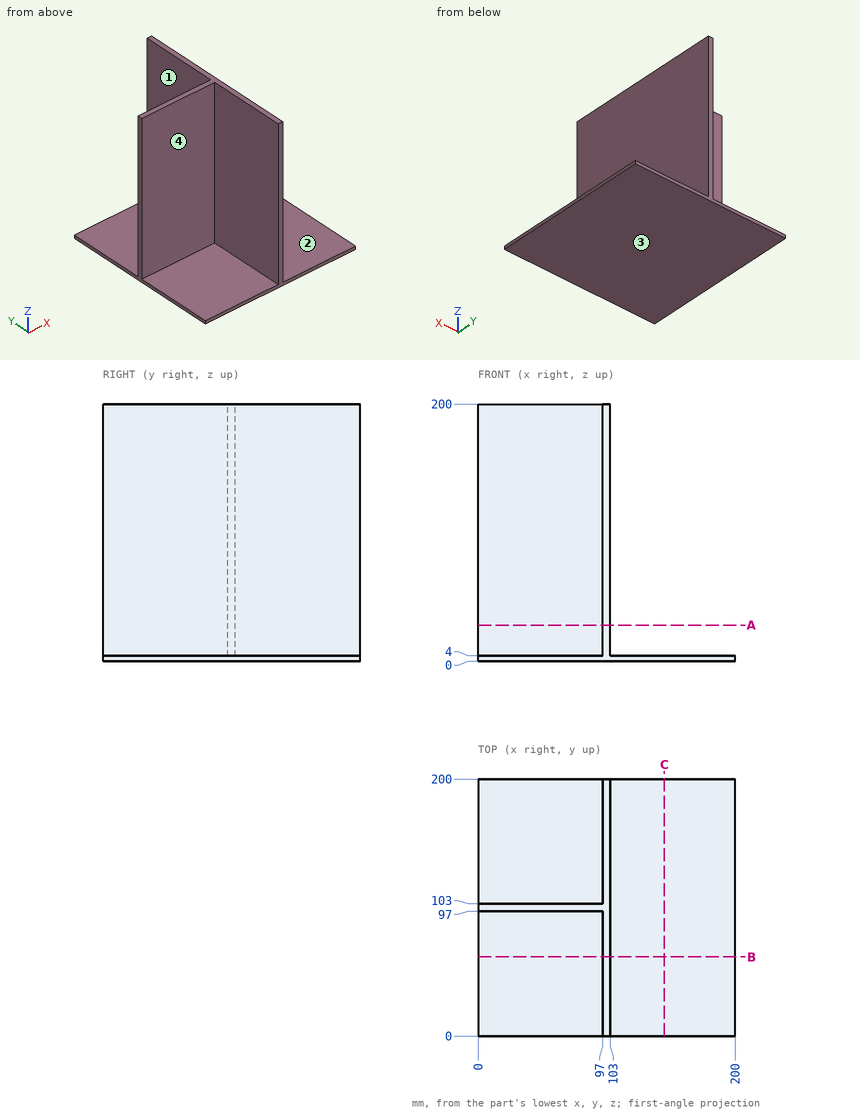
Job drawing, mm, ordinate dimensions from the low corner. One solid piece. A direction names the side the tool comes from. Coordinates: 2 decimals unless noted, no trailing zeros. Write each loop counter-clockwise with the first axis right and the second up, starting at its lowest first coordinate (ties: lowest second). Pieces come first, ordered by that corner, then holes. Notation, with made-up numbers: (67, 77.25) - (124, 77.25) arc R21 cw to (124, 96.25) - close; hole circle Ø6 at (86, -28). An arc over 180 degrees is marked (long way). Use a Markdown table: item, result. Add a question column.
Item 1: Band-saw the part on C-C, the plane x = 145. Give the cut face in (y, z), and give its area (3 significant figures).
Item 2: Drill centre lines: L1, parallel to Z at x = 39, y = 15; L2, parallel to X at y = 157, z = 140. Where is each one in solid material? Low to high. Write a range as from..to.
Item 3: Band-saw the part on A-A, the plane z = 28. Give the cut face in (x, y).
Item 4: Band-saw the part on B-B, the plane y = 61.5. Give the cut face in (x, z), and give its area (3 significant figures).
Item 5: Flat gauge pins, fed straight in: pin 1 (6 mm diameter, centred on x = 175, y = 100, fed in from -Z); pin 2 (12 mm diameter, centred on y = 173, z = 52, fed in from -X); pin 3 (6 mm diameter, centred on x = 21, y = 40, fed in from +Z); pin 4 (1.5 mm diameter, centred on y = 62, z = 150, fed in from +X). Where does each tip first touch, or does it go through?
Item 6: 3-axis set-ups, long thin cutter, end or side, ignore diameter. For the marked faces 1, 2, 3 and 4: which of +Z, -Z, +X, -X, +Y, -Y reach the whole face in a straight line?
Numbers:
| question | item | result |
|---|---|---|
| 1 | outline | (0, 0) - (200, 0) - (200, 4) - (0, 4) - close |
| 1 | area | 800 mm2 |
| 2 | L1 | 0..4 |
| 2 | L2 | 97..103 |
| 3 | outline | (0, 97) - (97, 97) - (97, 0) - (103, 0) - (103, 200) - (97, 200) - (97, 103) - (0, 103) - close |
| 4 | outline | (0, 0) - (200, 0) - (200, 4) - (103, 4) - (103, 200) - (97, 200) - (97, 4) - (0, 4) - close |
| 4 | area | 1,980 mm2 |
| 5 | pin 1 | z = 0 |
| 5 | pin 2 | x = 97 |
| 5 | pin 3 | z = 4 |
| 5 | pin 4 | x = 103 |
| 6 | face 1 | +Z, -X, +Y |
| 6 | face 2 | +Z, +X, +Y, -Y |
| 6 | face 3 | -Z, +X, -X, +Y, -Y |
| 6 | face 4 | +Z, -X, -Y |
